from build123d import *

# Parameters (mm, degrees)
F1_DEPTH = 3.175


# Not quite as in the source:
# - a length typed as a fraction of an inch, garbled in the dataset ("3 / 203.2 mm" for 3/8 in), is restored
# - a feature names something its author has since deleted; it is built from what else it names


with BuildPart() as f1:
    # F0 (on Front) → F1 (new body)
    with BuildSketch(Plane.XZ):
        with BuildLine():
            ThreePointArc((41.6017871916, 14.91), (41.5307431297, 15.6605366323), (41.3201345734, 16.3844126791))
            ThreePointArc((41.3201345734, 16.3844126791), (39.8492690362, 18.218900929), (37.6017871916, 18.91))
            Line((37.6017871916, 18.91), (19.6568542495, 18.91))
            Line((19.6568542495, 18.91), (28.870343186, 28.1234889365))
            ThreePointArc((28.870343186, 28.1234889365), (30.0382240231, 31.1237376944), (28.617137145, 34.0126735442))
            ThreePointArc((28.617137145, 34.0126735442), (25.870094428, 34.9482240231), (23.2134889365, 33.780343186))
            Line((23.2134889365, 33.780343186), (13.6523135737, 24.2191678232))
            ThreePointArc((13.6523135737, 24.2191678232), (10, 24.91), (6.3476864263, 24.2191678232))
            Line((6.3476864263, 24.2191678232), (-10.4648587405, 41.03171299))
            ThreePointArc((-10.4648587405, 41.03171299), (-12.3998071782, 42.1022210835), (-14.6078257676, 41.9811139245))
            ThreePointArc((-14.6078257676, 41.9811139245), (-15.418464559, 41.5920342359), (-16.12171299, 41.03171299))
            ThreePointArc((-16.12171299, 41.03171299), (-17.2932858653, 38.2032858653), (-16.12171299, 35.3748587405))
            Line((-16.12171299, 35.3748587405), (0.6908321768, 18.5623135737))
            ThreePointArc((0.6908321768, 18.5623135737), (0.1519224699, 16.6464817767), (0.003078879, 14.6618707992))
            Line((0.003078879, 14.6618707992), (-41.296146258, -4.5962741581))
            ThreePointArc((-41.296146258, -4.5962741581), (-43.1811508594, -6.4281956325), (-43.5221795995, -9.0345106623))
            ThreePointArc((-43.5221795995, -9.0345106623), (-43.4019791332, -9.4816883664), (-43.2309043592, -9.9119783532))
            ThreePointArc((-43.2309043592, -9.9119783532), (-40.9737537843, -11.9802757894), (-37.9152001641, -11.8467364544))
            Line((-37.9152001641, -11.8467364544), (3.3840249729, 7.4114085029))
            ThreePointArc((3.3840249729, 7.4114085029), (12.1643961394, 5.1470399288), (19.1651513899, 10.91))
            Line((19.1651513899, 10.91), (37.6017871916, 10.91))
            ThreePointArc((37.6017871916, 10.91), (40.4302143163, 12.0815728753), (41.6017871916, 14.91))
        make_face()
        with BuildLine():
            ThreePointArc((-40.5119809981, -8.644123568), (-40.5453658318, -7.8794851629), (-40.0282914728, -7.3151975192))
            ThreePointArc((-40.0282914728, -7.3151975192), (-39.2636530677, -7.2818126855), (-38.699365424, -7.7988870445))
            ThreePointArc((-38.699365424, -7.7988870445), (-38.6293772039, -8.0050656923), (-38.605673211, -8.2215053062))
            ThreePointArc((-38.605673211, -8.2215053062), (-38.7622817652, -8.7588049146), (-39.1830549493, -9.1278130933))
            ThreePointArc((-39.1830549493, -9.1278130933), (-39.9476933544, -9.161197927), (-40.5119809981, -8.644123568))
        make_face(mode=Mode.SUBTRACT)
        with BuildLine():
            ThreePointArc((-12.2932858653, 38.2032858653), (-12.3694063328, 37.8206024329), (-12.5861790841, 37.4961790841))
            ThreePointArc((-12.5861790841, 37.4961790841), (-13.2932858653, 37.2032858653), (-14.0003926465, 37.4961790841))
            ThreePointArc((-14.0003926465, 37.4961790841), (-14.2932858653, 38.2032858653), (-14.0003926465, 38.9103926465))
            ThreePointArc((-14.0003926465, 38.9103926465), (-13.2932858653, 39.2032858653), (-12.5861790841, 38.9103926465))
            ThreePointArc((-12.5861790841, 38.9103926465), (-12.3694063328, 38.5859692976), (-12.2932858653, 38.2032858653))
        make_face(mode=Mode.SUBTRACT)
        with BuildLine():
            ThreePointArc((14, 14.91), (13.3735657833, 12.7608015666), (11.690473047, 11.2847688519))
            ThreePointArc((11.690473047, 11.2847688519), (10, 10.91), (8.309526953, 11.2847688519))
            ThreePointArc((8.309526953, 11.2847688519), (6.060768988, 14.2154072893), (7.1715728753, 17.7384271247))
            ThreePointArc((7.1715728753, 17.7384271247), (10, 18.91), (12.8284271247, 17.7384271247))
            ThreePointArc((12.8284271247, 17.7384271247), (13.69551813, 16.4407337295), (14, 14.91))
        make_face(mode=Mode.SUBTRACT)
        with BuildLine():
            ThreePointArc((5.9466991411, 20.2133008589), (5.8515485567, 19.7349465684), (5.5805826176, 19.3294173824))
            ThreePointArc((5.5805826176, 19.3294173824), (3.8128156646, 19.3294173824), (3.8128156646, 21.0971843354))
            ThreePointArc((3.8128156646, 21.0971843354), (5.1750534316, 21.3681502745), (5.9466991411, 20.2133008589))
        make_face(mode=Mode.SUBTRACT)
        with BuildLine():
            ThreePointArc((16.3033008589, 20.2133008589), (15.6859842913, 19.2894213264), (14.5961940777, 19.5061940777))
            ThreePointArc((14.5961940777, 19.5061940777), (14.5961940777, 20.9204076401), (16.0104076401, 20.9204076401))
            ThreePointArc((16.0104076401, 20.9204076401), (16.2271803914, 20.5959842913), (16.3033008589, 20.2133008589))
        make_face(mode=Mode.SUBTRACT)
        with BuildLine():
            ThreePointArc((36.6017871916, 14.91), (37.6017871916, 15.91), (38.6017871916, 14.91))
            ThreePointArc((38.6017871916, 14.91), (37.6017871916, 13.91), (36.6017871916, 14.91))
        make_face(mode=Mode.SUBTRACT)
        with BuildLine():
            ThreePointArc((18.4246212025, 22.3346212025), (17.8073046348, 21.4107416699), (16.7175144213, 21.6275144213))
            ThreePointArc((16.7175144213, 21.6275144213), (16.7175144213, 23.0417279836), (18.1317279836, 23.0417279836))
            ThreePointArc((18.1317279836, 23.0417279836), (18.348500735, 22.7173046348), (18.4246212025, 22.3346212025))
        make_face(mode=Mode.SUBTRACT)
        with BuildLine():
            ThreePointArc((26.7490228424, 30.24480928), (26.0419160612, 29.9519160612), (25.33480928, 30.24480928))
            ThreePointArc((25.33480928, 30.24480928), (25.0419160612, 30.9519160612), (25.33480928, 31.6590228424))
            ThreePointArc((25.33480928, 31.6590228424), (26.0419160612, 31.9519160612), (26.7490228424, 31.6590228424))
            ThreePointArc((26.7490228424, 31.6590228424), (26.9657955937, 31.3345994936), (27.0419160612, 30.9519160612))
            ThreePointArc((27.0419160612, 30.9519160612), (26.9657955937, 30.5692326289), (26.7490228424, 30.24480928))
        make_face(mode=Mode.SUBTRACT)
    extrude(amount=F1_DEPTH)


solid = f1.part
The listing builds one solid part. Answer for the finished solid, in the listing's coordinates (mm). A direction names the side the tool comes from. Round coordinates to 2 decimals unless told otherwise and drop trailing zeros. Write each loop counter-clockwise with the first axis right and the second up, starting at its lowest first coordinate (ties: lowest second). Pieces come first, ordered by that corner, then holes. Notation, with made-up numbers: M 56,-3 L 107,-3 A29 ccw 107,19 Z; hole C 61,62.5 d1. An arc over 180 degrees is marked long. Write each question's results on one line, items separated by ' | '. Start each with the question number.
(1) Find the intervals of material crossed by line 1 (X direction, y = -2.2, z = 14.91); line 2 (Z direction, x = 26, y = -0.7); line 3 (X direction, y = -0.15, z = 19.5), in increasing order.
(2) The part is cut by section C-C, the plane x = 35. Write down the section's boundary in (y, z) (3 decimals), and give its area (3 significant figures).
(3) The part is cut by section B-B, the plane y = -0.8. Give the number of separate pieces and of enclosed holes in the cut face, and give its area (3 significant figures).
(4) The part is cut by section A-A, the plane x = -7. Write down the section's boundary in (y, z) (3 decimals), and give its area (3 significant figures).
(5) Determine the mould class of faces 1 (the flat face through (24.199, -1.565, 23.452)), 2 (the flat face through (-20.357, -1.565, 5.168)), 3 (the cylindrical face through (10.05, -1.57, 24.91)) for opening direction X: +X half, -X half, draft (parallel to the pull), parting line (faces both ways), or undercut.
(6) Each of these flat-tipped pins is pushed along its axis until it touches: P1, Ø1, axis at x = 33, y = -1.5, coming from the +Z side; P2, Ø1.5, axis at x = -26, y = -1.5, coming from the -Z side; P3, Ø1, axis at x = 6.5, y = -1.5, coming from the +Z side. Where does it stop, or does it pass through?
(7) The part is cut by section D-D, the plane x = -36. Write down the section's boundary in (y, z) (3 decimals), and give its area (3 significant figures).
(8) For faces 4 (the flat face through (-1.941, -1.565, 32.508)), 5 (the flat face through (28, -2, 10.91)), 6 (the flat face through (29, -2, 18.91)), determine the directions among +Z, -Z, +X, -X, +Y, -Y from which every point of the face is accessible in a straight line to the end or side of a thin tool.
Worked answers:
1) line 1: x = 0 to 6, 14 to 36.6, 38.6 to 41.6 | line 2: z = 10.91 to 18.91, 25.25 to 29.95, 31.95 to 34.95 | line 3: x = -0.25 to 3.67, 5.72 to 14.6, 16 to 20.25
2) outline: M -3.175,10.91 L 0,10.91 L 0,18.91 L -3.175,18.91 Z | area: 25.4 mm²
3) separate pieces: 1 | enclosed holes: 8 | area: 1,130 mm²
4) outline: M -3.175,2.569 L 0,2.569 L 0,11.396 L -3.175,11.396 Z; M -3.175,26.253 L 0,26.253 L 0,37.567 L -3.175,37.567 Z | area: 63.9 mm²
5) face 1: +X half | face 2: -X half | face 3: undercut
6) P1: stops at z = 18.91 | P2: stops at z = -6.64 | P3: stops at z = 24.57
7) outline: M -3.175,-10.954 L 0,-10.954 L 0,-2.127 L -3.175,-2.127 Z | area: 28.0 mm²
8) face 4: +Z, +Y, -Y | face 5: -Z, +X, +Y, -Y | face 6: +X, +Y, -Y
